Here's how the part is built. I have some questions about the finished solid (model axes, mm). A direction names the side the tool comes from. Coordinates: 2 decimals unless noted, no trailing zeros. Write each loop counter-clockwise with the first axis right and the second up, starting at its lowest first coordinate (ties: lowest second). Pieces come first, ordered by that corner, then holes. Notation, with made-up numbers: (74.5, 49) -> (112.5, 49) arc R25 cw to (112.5, 66) -> close; hole circle Ø8 at (75.5, 74.25). An arc over 180 degrees is marked (long way). Use a Markdown table: item, result. Add a question column.
Item 1: Imagine slicing it at A-A, the plane y = 45. Write out the boundary of the cut face in (x, z) (1 decimal).
Item 2: If I drill on line 1 along Y through (x, z) = (46, 132); line 2 along Z through (x, y) = (12.5, -3); line 3 along X through (y, z) = (100, 166), over which ranges is the centre line in solid material (lowest first)? Write a range as from..to.
Item 3: On a 3-axis mill with a long thin cutter (end or side, diameter ignored), from which of +Z, -Z, +X, -X, +Y, -Y can I reach the whole of each face in a straight line? I mean faces 5 (the flat face through (106, 90, 257.175)), 6 (the flat face through (5, 165.1, 174)), 7 (the cylindrical face through (27.095, -6.386, 28.793)). Say none if no direction works.
Item 4: Will these pins go through, and if not, where does the flat tip stop? pin 1 Ø6 at (y, z) = (151, 159.5) entering from -X; pin 2 Ø8 at (x, z) = (79.5, 208.5) entering from -Y.
Item 5: Imagine slicing it at B-B, the plane z = 106.5. Write out the boundary of the cut face in (x, y), and give its area (3 significant figures).
Item 6: Imagine slicing it at D-D, the plane z = 51.5. Write out the boundary of the cut face in (x, y).
Item 7: Imagine slicing it at C-C, the plane x = 46. Write out the boundary of the cut face in (y, z) (3 decimals), and give its area (3 significant figures).
Item 8: If we mould it in two halves opening along X, with no side actions, what happens to faces 1 (the flat face through (10.16, 90, 172)), 2 (the flat face through (214.312, 88, 127)), 3 (the flat face through (5, 90, 101.6)), 4 (the cylindrical face through (18.481, -6.386, 252.047))? For each: pulls with the +X half, pulls with the -X half, needs draft (parallel to the pull), parting line crosses it, or undercut.
Autodesk Inventor part; units mm, degrees
ref_plane "YZ Plane" through (0, 0, 0) normal (1, 0, 0) x (0, 1, 0)
ref_plane "XZ Plane" through (0, 0, 0) normal (0, 1, 0) x (-1, 0, 0)
ref_plane "XY Plane" through (0, 0, 0) normal (0, 0, 1) x (1, 0, 0)
sketch "Sketch1" plane through (0, 0, 0) normal (0, 0, 1) x (1, 0, 0)
  line L0 (0, 0) -> (214.3125, 0)
  line L1 (214.3125, 0) -> (214.3125, 177.8)
  line L2 (214.3125, 177.8) -> (0, 177.8)
  line L3 (0, 177.8) -> (0, 0)
  dimension "d0" = 214.3125
  dimension "d1" = 177.8
extrude "Extrusion1" add sketch "Sketch1" along normal blind 257.175
sketch "Sketch2" plane through (0, 0, 0) normal (0, -1, 0) x (1, 0, 0)
  line L0 (214.3125, 0) -> (214.3125, 257.175)
  line L1 (214.3125, 128.5875) -> (107.1562, 128.5875) construction
  line L2 (107.1562, 128.5875) -> (107.1562, 0) construction
  line L3 (214.3125, 257.175) -> (0, 257.175) construction
  line L4 (214.3125, 0) -> (214.3125, 257.175) construction
  line L5 (214.3125, 257.175) -> (214.3125, 239.649) construction
  line L6 (214.3125, 239.649) -> (196.9389, 239.649) construction
  circle A0 centre (196.9389, 239.649) radius 12.7
  circle A1 centre (196.9389, 17.526) radius 12.7
  line L7 (196.9389, 239.649) -> (11.3133, 239.649) construction
  circle A2 centre (21.2344, 239.649) radius 12.7
  line L8 (0, 0) -> (0, 257.175) construction
  circle A3 centre (21.2344, 17.526) radius 12.7
  dimension "d4" = 107.1562
  dimension "d6" = 17.526
  dimension "d7" = 17.3736
  dimension "d8" = 25.4
  dimension "d9" = 25.4
  dimension "d10" = 21.2344
extrude "Extrusion2" add sketch "Sketch2" along normal blind 25.4
fillet "Fillet1" radius 12.446 4 edges at (184.2389, -25.4, 239.649) (8.5344, -25.4, 239.649) (8.5344, -25.4, 17.526) (184.2389, -25.4, 17.526)
sketch "Sketch3" plane through (0, 0, 0) normal (-1, 0, 0) x (0, 0, 1)
  line L0 (257.175, 0) -> (257.175, 177.8)
  line L1 (257.175, 177.8) -> (257.175, 165.1)
  line L2 (257.175, 165.1) -> (244.475, 165.1)
  line L3 (0, 0) -> (101.6, 0)
  line L4 (101.6, 0) -> (101.6, 12.7)
  line L5 (244.475, 165.1) -> (101.6, 165.1)
  line L6 (101.6, 165.1) -> (101.6, 12.7)
  line L7 (101.6, 12.7) -> (244.475, 12.7)
  line L8 (244.475, 12.7) -> (244.475, 165.1)
  dimension "d14" = 12.7
  dimension "d15" = 12.7
  dimension "d16" = 101.6
  dimension "d17" = 12.7
extrude "Extrusion3" cut sketch "Sketch3" against normal blind 10.16
properties part number "PXie-1083"
Ans:
| question | item | result |
|---|---|---|
| 1 | outline | (0, 0) -> (214.3, 0) -> (214.3, 257.2) -> (0, 257.2) -> (0, 244.5) -> (10.2, 244.5) -> (10.2, 101.6) -> (0, 101.6) -> close |
| 2 | line 1 | y = 0..177.8 |
| 2 | line 2 | z = 8.31..26.75, 230.43..248.87 |
| 2 | line 3 | x = 10.16..214.31 |
| 3 | face 5 | +Z, +X, -X, +Y, -Y |
| 3 | face 6 | -X |
| 3 | face 7 | -Y |
| 4 | pin 1 | stops at x = 10.16 |
| 4 | pin 2 | stops at y = 0 |
| 5 | outline | (0, 0) -> (214.31, 0) -> (214.31, 177.8) -> (0, 177.8) -> (0, 165.1) -> (10.16, 165.1) -> (10.16, 12.7) -> (0, 12.7) -> close |
| 5 | area | 36,600 mm^2 |
| 6 | outline | (0, 0) -> (214.31, 0) -> (214.31, 177.8) -> (0, 177.8) -> close |
| 7 | outline | (0, 0) -> (177.8, 0) -> (177.8, 257.175) -> (0, 257.175) -> close |
| 7 | area | 45,700 mm^2 |
| 8 | face 1 | pulls with the -X half |
| 8 | face 2 | pulls with the +X half |
| 8 | face 3 | needs draft |
| 8 | face 4 | undercut |
